The listing builds one solid part. Answer for the finished solid, in the listing's coordinates (mm). A direction names the side the tool comes from. Give positions to 0.01 mm unless a question says otherwise; leave off trailing zeros. Order: outer loops, then holes, each group sorted by start corner. A loop starts at its lowest first (then second) coordinate and runs counter-clockwise, first axis right, second up. Notation, with made-up numbers: (29.25, 57) - (75.25, 57) arc R7 cw to (75.25, 67) - close; hole circle Ø9 at (39, -16). An arc over 180 degrees is marked (long way). Answer as CSV lines item,"result". Start each with the question number.
1. Determine the mould class of faces 4 (the cylindrical face through (-7.1, 2.54, 66.19)), 5 (the flat face through (57, 7, 40)), 6 (the flat face through (-40, 7, 57)) for opening direction Z: +Z half, -Z half, draft (parallel to the pull), parting line (faces both ways), or undercut.
2. Section D-D on z = -3 is taken. Give the vertices of the cut face in (x, y), and give its area (3 significant figures).
3. Section C-C on y = 7.75 is taken. Give the vertices of the cut face in (x, z), and give its area (3 significant figures).
4. Flat-ended cylindrical pins translate along their axes: pin 1 (3 mm diameter, centred on x = -48, z = -3, fed in from -Y); pin 2 (5.5 mm diameter, centred on y = 7, z = -59.5, fed in from +X); pin 3 (5.5 mm diameter, centred on y = 7.5, z = -56.5, fed in from -X); pin 4 (3 mm diameter, centred on y = 2.5, z = -23.5, fed in from -X). Find the tip coordinate at first contact, or state that the pin passes through.
5. Consider line 1 along Z through (x, y) = (-6.5, 4); line 2 along Z through (x, y) = (-36, 1.25); line 3 along Z through (x, y) = (-42.5, 1.5). Determine where each line is inside the solid, lowest interval first. Write a range as [from, to].
6. Section B-B on z = -21 is taken. Give the vertices of the cut face in (x, y).
7. Which of the six approach directions +Z, -Z, +X, -X, +Y, -Y give full straight-line access (tool end or side, diameter ignored) to faces 1 (the flat face through (-50, 4, 1)), 2 (the flat face through (57, 7, -40)), 3 (the flat face through (-40, 7, -57))?
8. Section A-A on x = 0 is taken. Give the vertices of the cut face in (y, z).
from build123d import *

# Parameters (mm, degrees)
SKETCH1_R           = 75
SKETCH1_W           = 100
SKETCH1_H           = 100
BOSS_EXTRUDE1_DEPTH = 5
SKETCH2_R           = 8
CUT_EXTRUDE1_DEPTH  = 10
BOSS_EXTRUDE2_DEPTH = 5


with BuildPart() as part:
    # Sketch1 → Boss-Extrude1 (new body)
    with BuildSketch(Plane(origin=(0, 0, 0), x_dir=(1, 0, 0), z_dir=(0, 1, 0))):
        with Locations(Location((0, 0, 0), (0, 0, 270))):
            Circle(SKETCH1_R)
        Rectangle(SKETCH1_W, SKETCH1_H, mode=Mode.SUBTRACT)
    extrude(amount=BOSS_EXTRUDE1_DEPTH)

    # Sketch2 → Cut-Extrude1 (cut)
    with BuildSketch(Plane(origin=(0, 5, 0), x_dir=(1, 0, 0), z_dir=(0, 1, 0))):
        with Locations(Location((-62.5, 0, 0), (0, 0, 270))):
            Circle(SKETCH2_R)
        with Locations(Location((0, 62.5, 0), (0, 0, 270))):
            Circle(SKETCH2_R)
        with Locations(Location((62.5, 0, 0), (0, 0, 270))):
            Circle(SKETCH2_R)
        with Locations(Location((0, -62.5, 0), (0, 0, 270))):
            Circle(SKETCH2_R)
    extrude(amount=-CUT_EXTRUDE1_DEPTH, mode=Mode.SUBTRACT)

    # Sketch3 → Boss-Extrude2 (add)
    with BuildSketch(Plane(origin=(0, 5, 0), x_dir=(1, 0, 0), z_dir=(0, 1, 0))):
        with BuildLine():
            Line((50, -50), (40, -50))
            Line((40, -50), (40, -63.442887702))
            ThreePointArc((40, -63.442887702), (53.033008589, -53.033008589), (63.442887702, -40))
            Line((63.442887702, -40), (50, -40))
            Line((50, -40), (50, -50))
        make_face()
        with BuildLine():
            Line((-40, -50), (-50, -50))
            Line((-50, -50), (-50, -40))
            Line((-50, -40), (-63.442887702, -40))
            ThreePointArc((-63.442887702, -40), (-53.033008589, -53.033008589), (-40, -63.442887702))
            Line((-40, -63.442887702), (-40, -50))
        make_face()
        with BuildLine():
            Line((-63.442887702, 40), (-50, 40))
            Line((-50, 40), (-50, 50))
            Line((-50, 50), (-40, 50))
            Line((-40, 50), (-40, 63.442887702))
            ThreePointArc((-40, 63.442887702), (-53.033008589, 53.033008589), (-63.442887702, 40))
        make_face()
        with BuildLine():
            Line((50, 50), (50, 40))
            Line((50, 40), (63.442887702, 40))
            ThreePointArc((63.442887702, 40), (53.033008589, 53.033008589), (40, 63.442887702))
            Line((40, 63.442887702), (40, 50))
            Line((40, 50), (50, 50))
        make_face()
    extrude(amount=BOSS_EXTRUDE2_DEPTH)


solid = part.part
Checks:
1,face 4,"undercut"
1,face 5,"undercut"
1,face 6,"draft"
2,outline,"(-74.94, 0) - (-69.92, 0) - (-69.92, 5) - (-74.94, 5) - close; (-55.08, 0) - (-50, 0) - (-50, 5) - (-55.08, 5) - close; (50, 0) - (55.08, 0) - (55.08, 5) - (50, 5) - close; (69.92, 0) - (74.94, 0) - (74.94, 5) - (69.92, 5) - close"
2,area,"101 mm²"
3,outline,"(-63.44, -40) arc R75 ccw to (-40, -63.44) - (-40, -50) - (-50, -50) - (-50, -40) - close; (-63.44, 40) - (-50, 40) - (-50, 50) - (-40, 50) - (-40, 63.44) arc R75 ccw to start; (40, -63.44) arc R75 ccw to (63.44, -40) - (50, -40) - (50, -50) - (40, -50) - close; (40, 50) - (50, 50) - (50, 40) - (63.44, 40) arc R75 ccw to (40, 63.44) - close"
3,area,"864 mm²"
4,pin 1,"passes through"
4,pin 2,"stops at x = 49.04"
4,pin 3,"stops at x = -52.31"
4,pin 4,"stops at x = -71.7"
5,line 1,"z = [-74.72, -67.16], [-57.84, -50], [50, 57.84], [67.16, 74.72]"
5,line 2,"z = [-65.8, -50], [50, 65.8]"
5,line 3,"z = [-61.8, -50], [50, 61.8]"
6,outline,"(-72, 0) - (-50, 0) - (-50, 5) - (-72, 5) - close; (50, 0) - (72, 0) - (72, 5) - (50, 5) - close"
7,face 1,"+Y, -Y"
7,face 2,"+X, -X, +Y"
7,face 3,"+Z, -Z, +Y"
8,outline,"(0, -75) - (5, -75) - (5, -70.5) - (0, -70.5) - close; (0, -54.5) - (5, -54.5) - (5, -50) - (0, -50) - close; (0, 50) - (5, 50) - (5, 54.5) - (0, 54.5) - close; (0, 70.5) - (5, 70.5) - (5, 75) - (0, 75) - close"
